Read the model definition and answer for the solid it produces. Units are mm, in the model's axes. A direction names the side the tool comes from. Give positions to 0.01 mm unless a question says otherwise; leave off trailing zeros. Loops run counter-clockwise (first coordinate to the right, second up) from the corner with the lowest first, then second, coordinate; pieces in that order, holes last. Notation, with made-up numbers: M 77,-6 L 116,-6 A33 cw 116,22 Z; hole C -23.5,87.5 d11. An arc over 180 degrees is marked long. Return JSON: item names as keys, results as strings. Group by question number.
Autodesk Inventor part; units mm, degrees
ref_plane "YZ Plane" through (0, 0, 0) normal (1, 0, 0) x (0, 1, 0)
ref_plane "XZ Plane" through (0, 0, 0) normal (0, 1, 0) x (-1, 0, 0)
ref_plane "XY Plane" through (0, 0, 0) normal (0, 0, 1) x (1, 0, 0)
sketch "Sketch1" plane through (0, 0, 0) normal (0, 1, 0) x (-1, 0, 0)
  line L0 (0, 0) -> (220.218, 0)
  line L1 (220.218, 0) -> (220.218, -267.97)
  line L2 (220.218, -267.97) -> (0, -267.97)
  line L3 (0, -267.97) -> (0, 0)
  circle A0 centre (110.109, -133.985) radius 57.15
  circle A1 centre (110.109, -133.985) radius 50.8
  line L4 (220.218, 0) -> (220.218, -25.4)
  line L5 (220.218, -133.985) -> (0, -133.985)
  line L6 (110.109, 0) -> (110.109, -267.97)
  line L7 (0, 0) -> (220.218, -267.97)
  line L8 (220.218, 0) -> (0, -267.97)
  line L9 (189.915, -36.8739) -> (146.3942, -89.8318)
  line L10 (220.218, -133.985) -> (167.259, -133.985)
  circle A2 centre (201.168, -248.92) radius 9.525
  circle A3 centre (201.168, -19.05) radius 9.525
  circle A4 centre (19.05, -248.92) radius 9.525
  circle A5 centre (19.05, -19.05) radius 9.525
  circle A6 centre (171.8873, -209.1593) radius 34.925
  circle A7 centre (48.3307, -209.1593) radius 34.925
  circle A8 centre (171.8873, -58.8107) radius 34.925
  circle A9 centre (48.3307, -58.8107) radius 34.925
  circle A10 centre (171.8873, -58.8107) radius 12.7
  circle A11 centre (171.8873, -209.1593) radius 12.7
  circle A12 centre (48.3307, -209.1593) radius 12.7
  circle A13 centre (48.3307, -58.8107) radius 12.7
  dimension "d0" = 220.218
  dimension "d1" = 267.97
  dimension "d11" = 114.3
  dimension "d12" = 101.6
  dimension "d40" = 69.85
  dimension "d41" = 25.4
  dimension "d42" = 25.4
extrude "Extrusion3" add sketch "Sketch1" along normal blind 40.64
extrude "Extrusion4" cut sketch "Sketch1" along normal blind 40.64 contours L6 L7 A1 | A1 L8 L6 | L5 L8 A1 | A1 L7 L5 | A1 L5 L8 | L7 A1 L6 | L5 A1 L7 | L6 A1 L8
sketch "Sketch3" plane through (0, 40.64, 0) normal (0, 1, 0) x (1, 0, 0)
  line L0 (0, 267.97) -> (-220.218, 267.97)
  line L1 (-220.218, 0) -> (0, 0)
  circle A0 centre (-110.109, 133.985) radius 57.15
  dimension "d21" = 114.3
extrude "Extrusion6" cut sketch "Sketch3" against normal blind 3.175
extrude "Extrusion8" cut sketch "Sketch1" along normal blind 87.3125 contours A5 L7 | L7 A5 | A3 L8 | L8 A3 | A4 L8 | L8 A4 | A2 L7 | L7 A2
extrude "Extrusion9" cut sketch "Sketch1" along normal blind 96.8375 contours A13 L7 | L7 A13 | A10 L8 | L8 A10 | A12 L8 | L8 A12 | A11 L7 | L7 A11
properties part number "Wash_Base_Middle"
1. Find section D-D (x = -72). Write down the section's boundary in (y, z) (3 decimals), and give its area (3 significant figures).
2. A flat-ended cylindrical pin translates along its axis: P1, Ø22, axis at x = -201.168, z = -248.92, coming from the +Y side. Find the tip coordinate at first contact, or state that the pin passes through.
3. Find section A-A (x = -19.05). Write down the section's boundary in (y, z) (3 decimals), and give its area (3 significant figures).
4. The mould has two halves that part along Z. Classify faces 3 (the flat face through (-112, 20, -267.97)), 4 (the flat face through (-220.218, 20, -132)), 5 (the cylindrical face through (-99.097, 18.47, -84.393)): +Z half, -Z half, draft (parallel to the pull), parting line (faces both ways), or undercut.
5. Find section B-B (z = -248.92). Write down the section's boundary in (x, y) (3 decimals), and give its area (3 significant figures).
6. Find section C-C (y = 23.5). State how many separate pieces and enclosed holes the cut face has, and give its area (3 significant figures).
7. For faces 1 (the cylindrical face through (-117.55, 39.07, -190.65)), 2 (the flat face through (0, 20, -136)), determine the directions among +Z, -Z, +X, -X, +Y, -Y from which every point of the face is accessible in a straight line to the end or side of a thin tool.
8. Straight lines are drawn through the part: line 1 along X through (y, z) = (16, -19); line 2 along X through (y, z) = (38, -18.5); line 3 along Z through (x, y) = (-45, 4.5). For each, find the intervals that lie inside material, in ascending order.
Result:
{
 "1": {"outline": "M 0,-267.97 L 40.64,-267.97 L 40.64,-176.574 L 37.465,-176.574 L 37.465,-167.576 L 0,-167.576 Z; M 0,-100.394 L 37.465,-100.394 L 37.465,-91.396 L 40.64,-91.396 L 40.64,0 L 0,0 Z", "area": "8,100 mm2"},
 "2": {"P1": "stops at y = 40.64"},
 "3": {"outline": "M 0,-267.97 L 40.64,-267.97 L 40.64,-258.445 L 0,-258.445 Z; M 0,-239.395 L 40.64,-239.395 L 40.64,-28.575 L 0,-28.575 Z; M 0,-9.525 L 40.64,-9.525 L 40.64,0 L 0,0 Z", "area": "9,340 mm2"},
 "4": {"face 3": "-Z half", "face 4": "draft", "face 5": "undercut"},
 "5": {"outline": "M -220.218,0 L -210.693,0 L -210.693,40.64 L -220.218,40.64 Z; M -191.643,0 L -28.575,0 L -28.575,40.64 L -191.643,40.64 Z; M -9.525,0 L 0,0 L 0,40.64 L -9.525,40.64 Z", "area": "7,400 mm2"},
 "6": {"separate pieces": "1", "enclosed holes": "9", "area": "47,700 mm2"},
 "7": {"face 1": "+Y", "face 2": "+Z, -Z, +X, +Y, -Y"},
 "8": {"line 1": "x = -220.22 to -210.69, -191.64 to -28.57, -9.53 to 0", "line 2": "x = -220.22 to -210.68, -191.66 to -28.56, -9.54 to 0", "line 3": "z = -267.97 to -221.41, -196.9 to -71.07, -46.56 to 0"}
}
